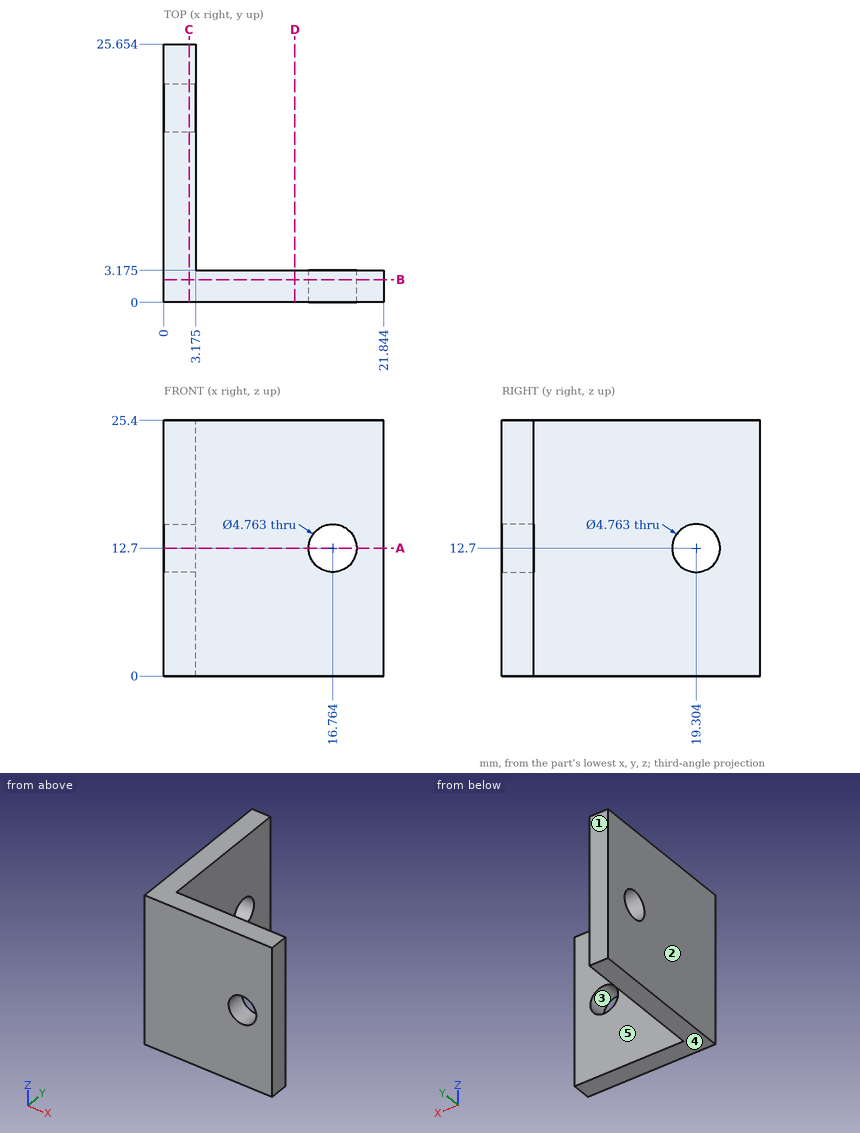
Drawing for the job (mm, zero at the part's lowest x, y, z). A direction names the side the tool comes from. Round coordinates to 2 decimals unless told otherwise and drop trailing zeros. Write each loop counter-clockwise with the first axis right and the second up, starting at its lowest first coordinate (ties: lowest second). Pieces come first, ordered by that corner, then holes. Notation, with made-up numbers: M -2.75,65.5 L 23.25,65.5 A26 cw 23.25,86.5 Z; hole C 69.5,31 d6. An arc over 180 degrees is marked long. Put each result on its own line as item: value.
Item 1: Cut at B-B (y = 2.25). List the corners of the cut face in (x, z) (1 decimal).
Responses:
outline: M 0,0 L 21.8,0 L 21.8,25.4 L 0,25.4 Z; hole C 16.8,12.7 d4.8
Item 2: Probe L1, parallel to Y at x = 2, z = 12.7 (1 decimal); L2, parallel to X at y = 2.55, z = 12.7 (1 decimal); L3, parallel to Y at x = 5.75, z = 23.5 (1 decimal). List the from-to ranges inside material, lowest first. Write a range as from..to.
Responses:
L1: 0..16.9, 21.7..25.7
L2: 0..14.4, 19.1..21.8
L3: 0..3.2
Item 3: Tool access for the marked faces 4 and 5: list every direction of +Z, -Z, +X, -X, +Y, -Y with a clear straight run to the whole face (end or side of a thin tool).
Responses:
face 4: -Z, +X, -X, +Y, -Y
face 5: +Z, -Z, +X, +Y
Item 4: Cut at A-A (z = 12.7). List the corners of the cut face in (x, y) (1 decimal).
Responses:
outline: M 0,0 L 14.4,0 L 14.4,3.2 L 3.2,3.2 L 3.2,16.9 L 0,16.9 Z; M 0,21.7 L 3.2,21.7 L 3.2,25.7 L 0,25.7 Z; M 19.1,0 L 21.8,0 L 21.8,3.2 L 19.1,3.2 Z
Item 5: Flat gauge pins, fed straight in: P1, Ø7.5, axis at y = 19.304, z = 12.7, coming from the -X side; P2, Ø5.5, axis at x = 13.5, z = 13.5, coming from the +Y side (1 decimal). Where does each tip first touch, or does it go through?
Responses:
P1: x = 0
P2: y = 3.2
Item 6: Cut at D-D (x = 13). List the corners of the cut face in (y, z) (1 decimal).
Responses:
outline: M 0,0 L 3.2,0 L 3.2,25.4 L 0,25.4 Z
Item 7: Mould opens along X. For the marked faces 1, 2 and 3 say: +X half, -X half, draft (parallel to the pull), parting line (faces both ways), or undercut.
Responses:
face 1: draft
face 2: -X half
face 3: undercut
Item 8: Cut at C-C (x = 2.5). List the corners of the cut face in (y, z) (1 decimal).
Responses:
outline: M 0,0 L 25.7,0 L 25.7,25.4 L 0,25.4 Z; hole C 19.3,12.7 d4.8
